Read the model definition and answer for the solid it produces. Units are mm, in the model's axes. A direction names the side the tool comes from. Give positions to 0.01 mm unless a question says otherwise; leave off trailing zeros. Order: outer loops, then holes, each group sorted by start corner. A loop starts at its lowest first (then second) coordinate and runs counter-clockwise, first axis right, second up. Notation, with made-up numbers: (43, 60) -> (89, 60) arc R23 cw to (89, 68) -> close; hole circle Ø1 at (-11.5, 40.5). An arc over 180 degrees is marked (long way). Answer as CSV lines item,"result". Start each with the question number.
1) The mould has two halves that part along Y. Classify faces 6 (the face through (36.397, 29.544, 5.916)), 7 (the face through (49.2, -14.9, 9.3)), 8 (the face through (37.933, 20.504, 3.057)), 9 (the face through (-48, -30, 6)): +Y half, -Y half, draft (parallel to the pull), parting line (faces both ways), or undercut.
2) Find section B-B (y = 0). Determine the outline of the cut face in (x, z), and give its area (3 significant figures).
3) Find section A-A (x = -52.5). Determine the outline of the cut face in (y, z), and give its area (3 significant figures).
4) Straight lines are drawn through the part: L1, parallel to Y at x = 52.5, z = 4; L2, parallel to Y at x = -52.5, z = 7.9; L3, parallel to X at y = 18, z = 4. For each, find the intervals that lie inside material, in ascending order. Write a range as from..to.
5) For faces 1 (the face through (-37, -24, 6.2)), 2 (the face through (29.597, 22.807, 6.084)), 3 (the face through (-52, -19, 6.5)), 4 (the face through (0, -48, 6.2)), 5 (the face through (61, 0, 6)), determine the directions among +Z, -Z, +X, -X, +Y, -Y from which every point of the face is accessible in a straight line to the end or side of a thin tool.
6) Find section D-D (y = 15). Determine the outline of the cut face in (x, z), and give its area (3 significant figures).
7) Flat-ended cylindrical pins translate along their axes: pin 1 Ø2.5 at (x, y) = (37.5, 20.5) entering from +Z; pin 2 Ø1 at (x, z) = (-4.5, 3) entering from -Y; pin 3 Ø4 at (x, z) = (21, 9.5) entering from +Y. Find the tip coordinate at first contact, or state that the pin passes through.
8) Find section C-C (x = 0). Determine the outline of the cut face in (y, z), and give its area (3 significant figures).
```python
from build123d import *

# Parameters (mm, degrees)
EXTRUDE_1_DEPTH              = 12
CUT_EXTRUDE_1_DEPTH          = 80.158069709
CUT_EXTRUDE_START            = -5.8
CUT_EXTRUDE_2_DEPTH          = 5.8
HOLE_WIZARD_4_5_4_5_1_D      = 4.5
HOLE_WIZARD_M64_1_D          = 72
HOLE_WIZARD_M6_1_D           = 6.6
HOLE_WIZARD_M6_1_CBORE_D     = 11
HOLE_WIZARD_M6_1_CBORE_DEPTH = 6.5
HOLE_WIZARD_M4_1_D           = 4.5
HOLE_WIZARD_M4_1_CBORE_D     = 8
HOLE_WIZARD_M4_1_CBORE_DEPTH = 5.8
FILLET_1_R                   = 1
FILLET_2_R                   = 5
FILLET_3_R                   = 7.5


with BuildPart() as part:
    # 草图1 → 凸台-拉伸1 (new body)
    with BuildSketch(Plane(origin=(0, 0, 0), x_dir=(-1, 0, 0), z_dir=(0, 0, -1))):
        with BuildLine():
            Line((61, -30), (61, 30))
            Line((61, 30), (-61, 30))
            Line((-61, 30), (-61, -30))
            Line((-61, -30), (-38.742741256, -30))
            ThreePointArc((-38.742741256, -30), (0, -49), (38.742741256, -30))
            Line((38.742741256, -30), (61, -30))
        make_face()
    extrude(amount=-EXTRUDE_1_DEPTH)

    # 草图2 → 切除-拉伸1 (cut, through all)
    with BuildSketch(Plane.XY.offset(12)):
        Polygon((-36.271415569, 30), (0, 0), (36.271415569, 30), align=None)
    extrude(amount=-CUT_EXTRUDE_1_DEPTH, mode=Mode.SUBTRACT)

    # 草图3 → 切除-拉伸2 (cut)
    with BuildSketch(Plane.XY.offset(12).offset(CUT_EXTRUDE_START)):
        with BuildLine():
            Line((4, -48.836461788), (4, -45))
            ThreePointArc((4, -45), (0, -41), (-4, -45))
            Line((-4, -45), (-4, -48.836461788))
            ThreePointArc((-4, -48.836461788), (0, -49), (4, -48.836461788))
        make_face()
    extrude(amount=CUT_EXTRUDE_2_DEPTH, mode=Mode.SUBTRACT)

    # Ø4.5 (4.5) 直径孔1 (through all)
    with Locations(Plane.XY.offset(6.2)):
        with Locations((0, -45)):
            Hole(HOLE_WIZARD_4_5_4_5_1_D / 2)

    # M64 间隙孔1 (through all)
    with Locations(Plane(origin=(0, 0, 0), x_dir=(-1, 0, 0), z_dir=(0, 0, -1))):
        with Locations((0, 0)):
            Hole(HOLE_WIZARD_M64_1_D / 2)

    # M6 六角头螺栓的柱形沉头孔1 (through all)
    with Locations(Plane(origin=(0, 0, 0), x_dir=(-1, 0, 0), z_dir=(0, 0, -1))):
        with Locations((-52.5, -15), (52.5, 15), (52.5, -15), (-52.5, 15)):
            CounterBoreHole(HOLE_WIZARD_M6_1_D / 2, HOLE_WIZARD_M6_1_CBORE_D / 2, HOLE_WIZARD_M6_1_CBORE_DEPTH)

    # M4 六角头机械螺钉的柱形沉头孔1 (through all)
    with Locations(Plane.XY.offset(12)):
        with Locations((38.97114317, 22.5), (38.97114317, -22.5), (-38.97114317, -22.5), (-38.97114317, 22.5)):
            CounterBoreHole(HOLE_WIZARD_M4_1_D / 2, HOLE_WIZARD_M4_1_CBORE_D / 2, HOLE_WIZARD_M4_1_CBORE_DEPTH)

    # 圆角1
    fillet_1_edges = [part.edges().sort_by_distance(p)[0] for p in [
        (4, -48.836461788, 9.1),
        (-4, -48.836461788, 9.1),
    ]]
    fillet(fillet_1_edges, radius=FILLET_1_R)

    # 圆角2
    fillet_2_edges = [part.edges().sort_by_distance(p)[0] for p in [
        (-38.742741256, -30, 6),
        (38.742741256, -30, 6),
        (61, -30, 6),
        (61, 30, 6),
        (-61, 30, 6),
        (-61, -30, 6),
        (-27.740852298, 22.944391772, 6),
        (27.740852298, 22.944391772, 6),
    ]]
    fillet(fillet_2_edges, radius=FILLET_2_R)

    # 圆角3
    fillet_3_edges = [part.edges().sort_by_distance(p)[0] for p in [
        (-36.271415569, 30, 6),
        (36.271415569, 30, 6),
    ]]
    fillet(fillet_3_edges, radius=FILLET_3_R)


solid = part.part
```
Findings below:
1,face 6,"+Y half"
1,face 7,"undercut"
1,face 8,"undercut"
1,face 9,"-Y half"
2,outline,"(-61, 0) -> (-36, 0) -> (-36, 12) -> (-61, 12) -> close; (36, 0) -> (61, 0) -> (61, 12) -> (36, 12) -> close"
2,area,"600 mm²"
3,outline,"(-30, 0) -> (-20.5, 0) -> (-20.5, 6.5) -> (-18.3, 6.5) -> (-18.3, 12) -> (-30, 12) -> close; (-11.7, 6.5) -> (-9.5, 6.5) -> (-9.5, 0) -> (9.5, 0) -> (9.5, 6.5) -> (11.7, 6.5) -> (11.7, 12) -> (-11.7, 12) -> close; (18.3, 6.5) -> (20.5, 6.5) -> (20.5, 0) -> (30, 0) -> (30, 12) -> (18.3, 12) -> close"
3,area,"504 mm²"
4,L1,"-30..-20.5, -9.5..9.5, 20.5..30"
4,L2,"-30..-18.3, -11.7..11.7, 18.3..30"
4,L3,"-61..-57.11, -47.89..-31.18, 31.18..47.89, 57.11..61"
5,face 1,"+Z"
5,face 2,"+Z, -Z"
5,face 3,"-Z"
5,face 4,"+Z, -Y"
5,face 5,"+Z, -Z, +X, +Y, -Y"
6,outline,"(-61, 0) -> (-58, 0) -> (-58, 6.5) -> (-55.8, 6.5) -> (-55.8, 12) -> (-61, 12) -> close; (-49.2, 6.5) -> (-47, 6.5) -> (-47, 0) -> (-32.73, 0) -> (-32.73, 12) -> (-49.2, 12) -> close; (32.73, 0) -> (47, 0) -> (47, 6.5) -> (49.2, 6.5) -> (49.2, 12) -> (32.73, 12) -> close; (55.8, 6.5) -> (58, 6.5) -> (58, 0) -> (61, 0) -> (61, 12) -> (55.8, 12) -> close"
6,area,"463 mm²"
7,pin 1,"z = 6.2"
7,pin 2,"y = -48.84"
7,pin 3,"y = -27.69"
8,outline,"(-49, 0) -> (-47.25, 0) -> (-47.25, 6.2) -> (-49, 6.2) -> close; (-42.75, 0) -> (-36, 0) -> (-36, 12) -> (-41, 12) -> (-41, 6.2) -> (-42.75, 6.2) -> close"
8,area,"81.7 mm²"
